Input: part model. Units: mm. Frame: model coordinates. Give positions to 0.01 mm unless a question says otherwise; leave off trailing zeros. Loops run counter-clockwise (first coordinate to the right, second up) from the corner with the lowest first, then second, coordinate; pieces in that order, holes last. Notation, with made-up numbers: (78.25, -11) - (120.25, -11) arc R17 ccw to (120.25, 21) - close; hole circle Ø4 at (68.25, -3). An arc over 180 degrees is marked (long way). Answer as a JSON object with one key per item and string values. Group by question number.
(1) Section query D-D (y = -2). Return loops of the section in (x, z), plus the area to 3 significant figures.
(2) Mould query, pull axis Z, two halves, no side actions, for faces 1 (the cylindrical face through (-23.655, -0.042, 0.479)), 2 (the flat face through (-11, 0, 3)), 3 (the flat face through (-11, -3, 0)). Classes: +Z half, -Z half, draft (parallel to the pull), parting line (faces both ways), or undercut.
(3) Section query C-C (y = 0). Return loops of the section in (x, z), plus the area to 3 significant figures.
(4) Pin query (flat end, axial travel): P1, Ø2, axis at x = -15, y = 0, coming from the +Z side. Return the tip coordinate at first contact, or that it passes through.
(5) Section query B-B (x = -15). Return loops of the section in (y, z).
(6) Material intervals for L1, parallel to Y at x = 0, z = -1.4; L2, parallel to X at y = 0.25, z = 2.75, sorted ascending.
(7) Section query A-A (z = 0). Return loops of the section in (x, y), plus the area to 3 significant figures.
```python
from build123d import *

# Parameters (mm, degrees)
SKETCH_2_W         = 28.5
SKETCH_2_H         = 6
SKETCH_2_R         = 0.5
EXTRUDE_1_DEPTH    = 3
HOLE_WIZARD_M3_1_D = 2.5
HOLE_WIZARD_M3_2_D = 2.5
CHAMFER_1_SIZE     = 0.5


with BuildPart() as part:
    # 草图2 → 凸台-拉伸1 (new body, symmetric)
    with BuildSketch(Plane.XY):
        with Locations((-11.25, 0)):
            Rectangle(SKETCH_2_W, SKETCH_2_H)
        with Locations((-15, 0)):
            Circle(SKETCH_2_R, mode=Mode.SUBTRACT)
        Circle(SKETCH_2_R, mode=Mode.SUBTRACT)
    extrude(amount=EXTRUDE_1_DEPTH, both=True)

    # M3 螺纹孔1 (through all)
    with Locations(Plane.XY.offset(3)):
        with Locations((0, 0), (-15, 0)):
            Hole(HOLE_WIZARD_M3_1_D / 2)

    # M3 螺纹孔2 (through all)
    with Locations(Plane(origin=(0, 3, 0), x_dir=(1, 0, 0), z_dir=(0, 1, 0))):
        with Locations((-7.5, 0), (-22.5, 0)):
            Hole(HOLE_WIZARD_M3_2_D / 2)

    # 倒角1
    chamfer_1_edges = [part.edges().sort_by_distance(p)[0] for p in [
        (-11.25, -3, 3),
        (3, 0, 3),
        (-11.25, 3, 3),
        (3, 0, -3),
        (-11.25, -3, -3),
        (-25.5, 0, -3),
        (-11.25, 3, -3),
        (-25.5, 0, 3),
        (3, 3, 0),
        (3, -3, 0),
        (-25.5, -3, 0),
        (-25.5, 3, 0),
    ]]
    chamfer(chamfer_1_edges, length=CHAMFER_1_SIZE)


solid = part.part
```
Recorded:
{
 "1": {"outline": "(-25.5, -2.5) - (-25, -3) - (2.5, -3) - (3, -2.5) - (3, 2.5) - (2.5, 3) - (-25, 3) - (-25.5, 2.5) - close; hole circle Ø2.5 at (-22.5, 0); hole circle Ø2.5 at (-7.5, 0)", "area": "161 mm^2"},
 "2": {"face 1": "undercut", "face 2": "+Z half", "face 3": "draft"},
 "3": {"outline": "(-25.5, -2.5) - (-25, -3) - (-16.25, -3) - (-16.25, 3) - (-25, 3) - (-25.5, 2.5) - close; (-13.75, -3) - (-1.25, -3) - (-1.25, 3) - (-13.75, 3) - close; (1.25, -3) - (2.5, -3) - (3, -2.5) - (3, 2.5) - (2.5, 3) - (1.25, 3) - close; hole circle Ø2.5 at (-22.5, 0); hole circle Ø2.5 at (-7.5, 0)", "area": "131 mm^2"},
 "4": {"P1": "passes through"},
 "5": {"outline": "(-3, -2.5) - (-2.5, -3) - (-1.25, -3) - (-1.25, 3) - (-2.5, 3) - (-3, 2.5) - close; (1.25, -3) - (2.5, -3) - (3, -2.5) - (3, 2.5) - (2.5, 3) - (1.25, 3) - close"},
 "6": {"L1": "y = -3 to -1.25, 1.25 to 3", "L2": "x = -25.25 to -16.22, -13.78 to -1.22, 1.22 to 2.75"},
 "7": {"outline": "(-25.5, -2.5) - (-25, -3) - (-23.75, -3) - (-23.75, 3) - (-25, 3) - (-25.5, 2.5) - close; (-21.25, -3) - (-8.75, -3) - (-8.75, 3) - (-21.25, 3) - close; (-6.25, -3) - (2.5, -3) - (3, -2.5) - (3, 2.5) - (2.5, 3) - (-6.25, 3) - close; hole circle Ø2.5 at (-15, 0); hole circle Ø2.5 at (0, 0)", "area": "131 mm^2"}
}
